Geometry: final body of the model. Coordinates: model frame, mm. A direction names the side the tool comes from. Coordinates: 2 decimals unless noted, no trailing zeros. Order: outer loops, then holes, each group sorted by start corner. A loop starts at its lowest first (then second) coordinate and runs counter-clockwise, first axis right, second up. Notation, with made-up numbers: M 87,19 L 120,19 A14 ccw 120,28 Z; hole C 47,85 d6. An arc over 180 degrees is marked long. Write item = value, one per line.
from build123d import *

# Parameters (mm, degrees)
SKETCH2_W           = 133.35
SKETCH2_H           = 160.866666666
SKETCH2_W_2         = 107.95
SKETCH2_H_2         = 135.466666666
BOSS_EXTRUDE1_DEPTH = 12.7
CUT_EXTRUDE1_DEPTH  = 6.35
CHAMFER1_SIZE       = 0.635
CHAMFER3_SIZE       = 3.81
SKETCH5_W           = 8.89
SKETCH5_H           = 11.43
CUT_EXTRUDE2_DEPTH  = 10.16
SKETCH6_W           = 8.89
SKETCH6_H           = 11.43
CUT_EXTRUDE3_DEPTH  = 10.16
CHAMFER4_SIZE       = 3.175
SKETCH7_W           = 12.7
SKETCH7_H           = 124.46
BOSS_EXTRUDE2_DEPTH = 2.286
CHAMFER5_SIZE       = 2.286


with BuildPart() as part:
    # Sketch2 → Boss-Extrude1 (new body)
    with BuildSketch(Plane(origin=(0, 0, 0), x_dir=(1, 0, 0), z_dir=(0, 1, 0))):
        Rectangle(SKETCH2_W, SKETCH2_H)
        Rectangle(SKETCH2_W_2, SKETCH2_H_2, mode=Mode.SUBTRACT)
    extrude(amount=BOSS_EXTRUDE1_DEPTH)

    # Sketch4 → Cut-Extrude1 (cut)
    with BuildSketch(Plane(origin=(0, 0, 0), x_dir=(1, 0, 0), z_dir=(0, 1, 0))):
        Polygon((-63.5, 76.2), (-60.325, 79.375), (-57.15, 76.2), (-60.325, 73.025), align=None)
        Polygon((-52.916666667, 76.2), (-49.741666667, 79.375), (-46.566666667, 76.2), (-49.741666667, 73.025), align=None)
        Polygon((57.15, 76.2), (60.325, 79.375), (63.5, 76.2), (60.325, 73.025), align=None)
        Polygon((57.15, -76.2), (60.325, -73.025), (63.5, -76.2), (60.325, -79.375), align=None)
        Polygon((-52.916666667, -76.2), (-49.741666667, -73.025), (-46.566666667, -76.2), (-49.741666667, -79.375), align=None)
        Polygon((-63.5, -76.2), (-60.325, -73.025), (-57.15, -76.2), (-60.325, -79.375), align=None)
    extrude(amount=CUT_EXTRUDE1_DEPTH, mode=Mode.SUBTRACT)

    # Chamfer1
    chamfer1_edges = [part.edges().sort_by_distance(p)[0] for p in [
        (-61.9125, 0, 77.7875),
        (-58.7375, 0, 77.7875),
        (-58.7375, 0, 74.6125),
        (-61.9125, 0, 74.6125),
        (-61.9125, 6.35, 77.7875),
        (-58.7375, 6.35, 77.7875),
        (-58.7375, 6.35, 74.6125),
        (-61.9125, 6.35, 74.6125),
        (-51.329166667, 0, 77.7875),
        (-52.916666667, 3.175, 76.2),
        (-48.154166667, 0, 77.7875),
        (-48.154166667, 0, 74.6125),
        (-51.329166667, 0, 74.6125),
        (-49.741666667, 3.175, 73.025),
        (-51.329166667, 6.35, 77.7875),
        (-48.154166667, 6.35, 77.7875),
        (-48.154166667, 6.35, 74.6125),
        (-51.329166667, 6.35, 74.6125),
        (58.7375, 0, 77.7875),
        (61.9125, 0, 77.7875),
        (61.9125, 0, 74.6125),
        (58.7375, 0, 74.6125),
        (58.7375, 6.35, 77.7875),
        (61.9125, 6.35, 77.7875),
        (61.9125, 6.35, 74.6125),
        (58.7375, 6.35, 74.6125),
        (58.7375, 0, -74.6125),
        (61.9125, 0, -74.6125),
        (61.9125, 0, -77.7875),
        (58.7375, 0, -77.7875),
        (58.7375, 6.35, -74.6125),
        (61.9125, 6.35, -74.6125),
        (61.9125, 6.35, -77.7875),
        (58.7375, 6.35, -77.7875),
        (-51.329166667, 0, -74.6125),
        (-48.154166667, 0, -74.6125),
        (-48.154166667, 0, -77.7875),
        (-51.329166667, 0, -77.7875),
        (-51.329166667, 6.35, -74.6125),
        (-48.154166667, 6.35, -74.6125),
        (-48.154166667, 6.35, -77.7875),
        (-51.329166667, 6.35, -77.7875),
        (-61.9125, 0, -74.6125),
        (-58.7375, 0, -74.6125),
        (-58.7375, 0, -77.7875),
        (-61.9125, 0, -77.7875),
        (-61.9125, 6.35, -74.6125),
        (-58.7375, 6.35, -74.6125),
        (-58.7375, 6.35, -77.7875),
        (-61.9125, 6.35, -77.7875),
    ]]
    chamfer(chamfer1_edges, length=CHAMFER1_SIZE)

    # Chamfer3
    chamfer3_edges = [part.edges().sort_by_distance(p)[0] for p in [
        (0, 12.7, -80.433333333),
        (0, 12.7, 80.433333333),
    ]]
    chamfer(chamfer3_edges, length=CHAMFER3_SIZE)

    # Sketch5 → Cut-Extrude2 (cut)
    with BuildSketch(Plane.XY.offset(80.433333333)):
        with Locations((-38.0365, 6.985)):
            Rectangle(SKETCH5_W, SKETCH5_H)
        with Locations((48.641, 6.985)):
            Rectangle(SKETCH5_W, SKETCH5_H)
    extrude(amount=-CUT_EXTRUDE2_DEPTH, mode=Mode.SUBTRACT)

    # Sketch6 → Cut-Extrude3 (cut)
    with BuildSketch(Plane(origin=(0, 0, -80.433333333), x_dir=(-1, 0, 0), z_dir=(0, 0, -1))):
        with Locations((38.0365, 6.985)):
            Rectangle(SKETCH6_W, SKETCH6_H)
        with Locations((-48.641, 6.985)):
            Rectangle(SKETCH6_W, SKETCH6_H)
    extrude(amount=-CUT_EXTRUDE3_DEPTH, mode=Mode.SUBTRACT)

    # Chamfer4
    chamfer4_edges = [part.edges().sort_by_distance(p)[0] for p in [
        (53.975, 0, 0),
        (0, 0, -67.733333333),
        (0, 0, 67.733333333),
    ]]
    chamfer(chamfer4_edges, length=CHAMFER4_SIZE)

    # Sketch7 → Boss-Extrude2 (add)
    with BuildSketch(Plane(origin=(0, 12.7, 0), x_dir=(1, 0, 0), z_dir=(0, 1, 0))):
        with Locations((60.325, 0)):
            Rectangle(SKETCH7_W, SKETCH7_H)
    extrude(amount=BOSS_EXTRUDE2_DEPTH)

    # Chamfer5
    chamfer5_edges = [part.edges().sort_by_distance(p)[0] for p in [
        (60.325, 14.986, 62.23),
        (60.325, 14.986, -62.23),
    ]]
    chamfer(chamfer5_edges, length=CHAMFER5_SIZE - 0.0001)  # a hair under: the kernel refuses the full size


solid = part.part
1) Line query: L1, parallel to X at y = 5.25, z = -7 (3 decimals); L2, parallel to Z at x = 51, y = 7; L3, parallel to Z at x = 24, y = 3.75. Output: solid intervals per line, ascending.
Numbers:
L1 = -66.675 to -53.975, 53.975 to 66.675
L2 = -70.27 to -67.73, 67.73 to 70.27
L3 = -80.43 to -67.73, 67.73 to 80.43
2) Section B-B, the plane x = 33. Return loops of the section in (y, z) (3 decimals).
Numbers:
outline = M 0,-80.433 L 8.89,-80.433 L 12.7,-76.623 L 12.7,-67.733 L 3.175,-67.733 L 0,-70.908 Z; M 0,70.908 L 3.175,67.733 L 12.7,67.733 L 12.7,76.623 L 8.89,80.433 L 0,80.433 Z
3) Section A-A, the plane z = -55. Return loops of the section in (x, y) (3 decimals).
Numbers:
outline = M -66.675,0 L -53.975,0 L -53.975,12.7 L -66.675,12.7 Z; M 53.975,3.175 L 57.15,0 L 66.675,0 L 66.675,14.986 L 53.975,14.986 Z
4) Set-up query: faces 4 (the face through (-47.9, 0.32, 77.98)), 5 (the face through (44.196, 7, 75)), 6 (the face through (-1, 8, -67.733)). Return all of +Z, -Z, +X, -X, +Y, -Y with unobstructed straight access to the full face (end or side cutting, diameter ignored); none if empty.
Numbers:
face_4 = -Y
face_5 = +Z, +Y
face_6 = +Y, -Y
5) Section D-D, the plane x = 49. Return loops of the section in (y, z) (3 decimals).
Numbers:
outline = M 0,-80.433 L 1.27,-80.433 L 1.27,-70.273 L 12.7,-70.273 L 12.7,-67.733 L 3.175,-67.733 L 0,-70.908 Z; M 0,70.908 L 3.175,67.733 L 12.7,67.733 L 12.7,70.273 L 1.27,70.273 L 1.27,80.433 L 0,80.433 Z
6) Section C-C, the plane y = 11. Return loops of the section in (x, z) (1 decimal).
Numbers:
outline = M -66.7,-78.3 L -42.5,-78.3 L -42.5,-70.3 L -33.6,-70.3 L -33.6,-78.3 L 44.2,-78.3 L 44.2,-70.3 L 53.1,-70.3 L 53.1,-78.3 L 66.7,-78.3 L 66.7,78.3 L 53.1,78.3 L 53.1,70.3 L 44.2,70.3 L 44.2,78.3 L -33.6,78.3 L -33.6,70.3 L -42.5,70.3 L -42.5,78.3 L -66.7,78.3 Z; hole M -54,-67.7 L 54,-67.7 L 54,67.7 L -54,67.7 Z
7) Pin query (flat end, axial travel): pin 1 (2.5 mm diameter, centred on x = -49.5, z = 75.5, fed in from -Y); pin 2 (3.5 mm diameter, centred on x = -59.5, z = 76.5, fed in from -Y); pin 3 (1.4 mm diameter, centred on x = 60.5, z = -77, fed in from -Y). Return the tip coordinate at first contact, or that it passes through.
Numbers:
pin_1 = 6.04
pin_2 = 0.33
pin_3 = 6.35
8) Mould query, pull axis Z, two halves, no side actions, for faces 1 (the face through (58.488, 0.322, -77.98)), 2 (the face through (-60, 6.35, -76)), 3 (the face through (53.086, 7, -75)). Classes: pulls with the +Z half, pulls with the -Z half, needs draft (parallel to the pull), parting line crosses it, or undercut.
Numbers:
face_1 = undercut
face_2 = undercut
face_3 = needs draft
